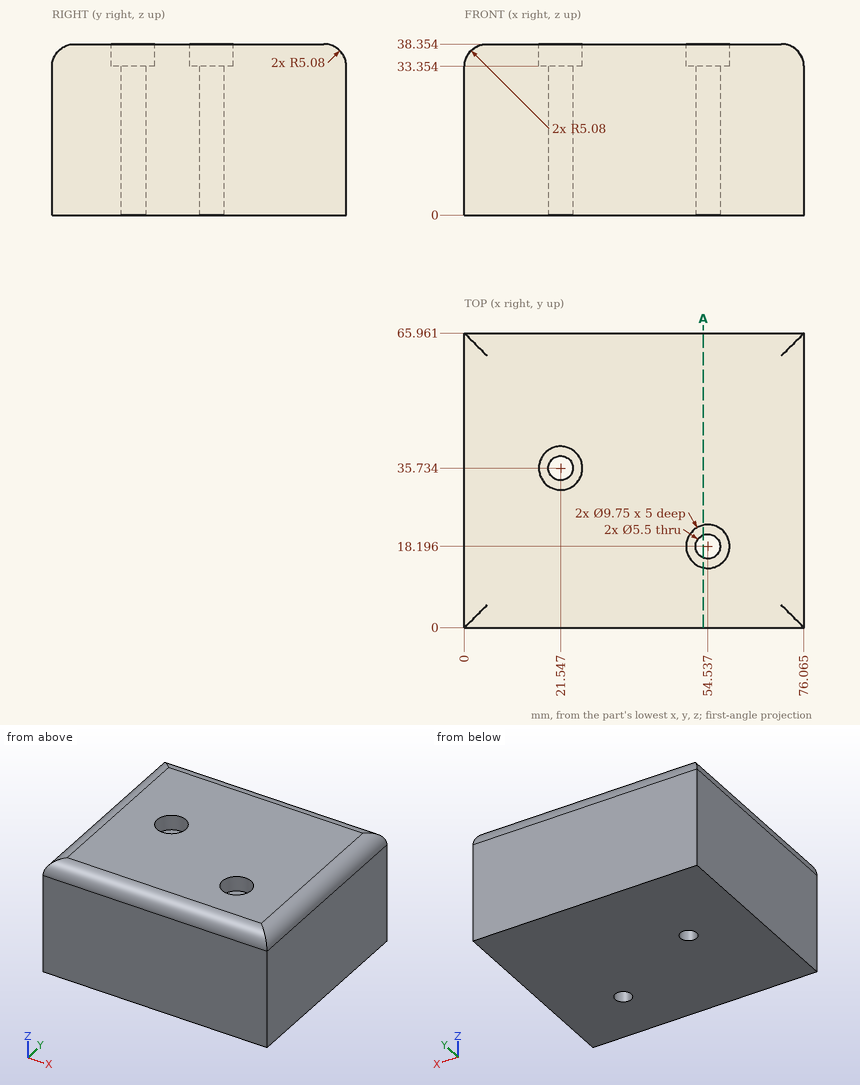
For this review, use the dimensioned drawing (mm, ordinates from the lowest corner) and the shaded views. Give positions to 0.01 mm unless a question says otherwise; leave off trailing zeros. Order: outer loops, then holes, each group sorted by start corner. A loop starts at its lowest first (then second) coordinate and runs counter-clockwise, first axis right, second up.
1. To check wall thickness, follow L1, parallel to X at y = 36, z = 13 (1 decimal); L2, parallel to X at y = 18, z = 16 (1 decimal); L3, parallel to Z at x = 26, y = 5. State the ranges of each line that lie inside material, in increasing order.
Solution:
L1: x = 0 to 18.8, 24.3 to 76.1
L2: x = 0 to 51.8, 57.3 to 76.1
L3: z = 0 to 38.35
2. For pin 1 Ø8 at (x, y) = (55.5, 16.5) entering from +Z; pin 2 Ø9 at (x, y) = (54.54, 18.2) entering from +Z, all flat-tipped, find the tip position at first contact; note any pin that passes through.
Solution:
pin 1: stops at z = 38.35
pin 2: stops at z = 33.35
3. Add section A-A, the plane x = 53.5. State the section outline as (y, z) points, then the cut area to 3 significant figures.
Solution:
outline: (0, 0) - (15.65, 0) - (15.65, 33.35) - (13.43, 33.35) - (13.43, 38.35) - (5.08, 38.35) arc R5.08 ccw to (0, 33.27) - close; (20.74, 0) - (65.96, 0) - (65.96, 33.27) arc R5.08 ccw to (60.88, 38.35) - (22.96, 38.35) - (22.96, 33.35) - (20.74, 33.35) - close
area: 2,300 mm2
